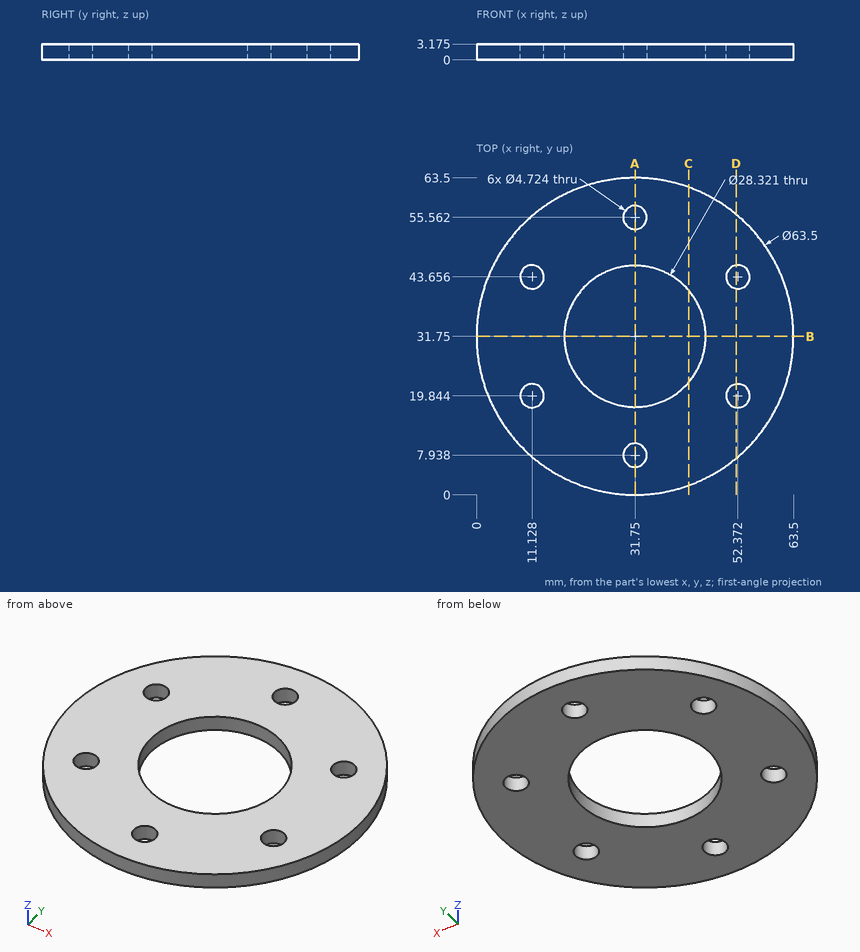
Could you check a few things on this drawing? It's one solid part, dimensions in mm from its lowest x, y, z. Coordinates: 2 decimals unless noted, no trailing zeros. Order: outer loops, then holes, each group sorted by start corner. A loop starts at its lowest first (then second) coordinate and runs counter-clockwise, first axis right, second up. Notation, with made-up numbers: M -12,-6 L 22,-6 A34 cw 22,32 Z; hole C 36.25,74.5 d1. An arc over 180 degrees is marked long. Answer as CSV lines item,"result".
(1) I'm going to push flat-ended pins straight in: pin 1 (1 mm diameter, centred on x = 36, z = 2.5, fed in from +Y); pin 2 (4.5 mm diameter, centred on x = 11.13, y = 19.84, fed in from +Z); pin 3 (1.5 mm diameter, centred on x = 24.5, z = 2.5, fed in from +Y). Where does each tip first touch, or does it pass through?
Geometry check:
pin 1,"y = 63.28"
pin 2,"through"
pin 3,"y = 62.83"
(2) Suppose I cut it at D-D on x = 52. Please give me the cut outline in (y, z) (1 decimal).
Geometry check:
outline,"M 7.3,0 L 17.5,0 L 17.5,3.2 L 7.3,3.2 Z; M 22.2,0 L 41.3,0 L 41.3,3.2 L 22.2,3.2 Z; M 46,0 L 56.2,0 L 56.2,3.2 L 46,3.2 Z"
(3) Suppose I cut it at A-A on x = 31.75. Please give me the cut outline in (y, z) (1 decimal).
Geometry check:
outline,"M 0,0 L 5.6,0 L 5.6,3.2 L 0,3.2 Z; M 10.3,0 L 17.6,0 L 17.6,3.2 L 10.3,3.2 Z; M 45.9,0 L 53.2,0 L 53.2,3.2 L 45.9,3.2 Z; M 57.9,0 L 63.5,0 L 63.5,3.2 L 57.9,3.2 Z"
(4) Suppose I cut it at C-C on x = 42.5. Please give me the cut outline in (y, z) (1 decimal).
Geometry check:
outline,"M 1.9,0 L 22.5,0 L 22.5,3.2 L 1.9,3.2 Z; M 41,0 L 61.6,0 L 61.6,3.2 L 41,3.2 Z"
(5) Please list where these lines run through material, in increasing order: L1, parallel to Y at x = 31.75, z = 1.5 (1 decimal); L2, parallel to Y at x = 12.5, z = 1.95 (1 decimal); L3, parallel to Y at x = 9.5, z = 2.9 (1 decimal).
Geometry check:
L1,"0 to 5.6, 10.3 to 17.6, 45.9 to 53.2, 57.9 to 63.5"
L2,"6.5 to 17.9, 21.8 to 41.7, 45.6 to 57"
L3,"9.1 to 18.1, 21.6 to 41.9, 45.4 to 54.4"
(6) Suppose I cut it at B-B on y = 31.75. Please give me the cut outline in (x, z) (1 decimal).
Geometry check:
outline,"M 0,0 L 17.6,0 L 17.6,3.2 L 0,3.2 Z; M 45.9,0 L 63.5,0 L 63.5,3.2 L 45.9,3.2 Z"
